```python
from build123d import *

# Parameters (mm, degrees)
SKETCH1_R           = 10.5
SKETCH1_R_2         = 9
BOSS_EXTRUDE1_DEPTH = 38.3
SKETCH2_R           = 1
SKETCH2_R_2         = 9
BOSS_EXTRUDE2_DEPTH = 1.5
FILLET1_R           = 0.5
SKETCH10_R          = 7.65
CUT_EXTRUDE1_DEPTH  = 46.293682625
SKETCH15_R          = 20.755300819
CUT_EXTRUDE3_DEPTH  = 17.5


with BuildPart() as part:
    # Sketch1 → Boss-Extrude1 (new body)
    with BuildSketch(Plane(origin=(0, 0, 0), x_dir=(1, 0, 0), z_dir=(0, 1, 0))):
        with Locations(Location((0, 0, 0), (0, 0, 270))):
            Circle(SKETCH1_R)
        with Locations(Location((0, 0, 0), (0, 0, 270))):
            Circle(SKETCH1_R_2, mode=Mode.SUBTRACT)
    extrude(amount=BOSS_EXTRUDE1_DEPTH)

    # Sketch2 → Boss-Extrude2 (add)
    with BuildSketch(Plane(origin=(0, 38.3, 0), x_dir=(1, 0, 0), z_dir=(0, 1, 0))):
        with BuildLine():
            Line((-3, -12.1346611), (-3, -12.5))
            ThreePointArc((-3, -12.5), (0, -15.5), (3, -12.5))
            Line((3, -12.5), (3, -12.1346611))
            ThreePointArc((3, -12.1346611), (6.25, -10.825317547), (9.008924778, -8.665406761))
            Line((9.008924778, -8.665406761), (9.325317547, -8.848076211))
            ThreePointArc((9.325317547, -8.848076211), (13.423393759, -7.75), (12.325317547, -3.651923789))
            Line((12.325317547, -3.651923789), (12.008924778, -3.469254338))
            ThreePointArc((12.008924778, -3.469254338), (12.393060767, -1.631577403), (12.497639685, 0.24290392))
            Line((12.497639685, 0.24290392), (12.850529964, 0.337460585))
            ThreePointArc((12.850529964, 0.337460585), (14.971850307, 4.011695199), (11.297615693, 6.133015543))
            Line((11.297615693, 6.133015543), (10.944725414, 6.038458877))
            ThreePointArc((10.944725414, 6.038458877), (7.609517863, 9.916916754), (3, 12.1346611))
            Line((3, 12.1346611), (3, 12.5))
            ThreePointArc((3, 12.5), (0, 15.5), (-3, 12.5))
            Line((-3, 12.5), (-3, 12.1346611))
            ThreePointArc((-3, 12.1346611), (-7.609517863, 9.916916754), (-10.944725414, 6.038458877))
            Line((-10.944725414, 6.038458877), (-11.297615693, 6.133015543))
            ThreePointArc((-11.297615693, 6.133015543), (-14.971850307, 4.011695199), (-12.850529964, 0.337460585))
            Line((-12.850529964, 0.337460585), (-12.497639685, 0.24290392))
            ThreePointArc((-12.497639685, 0.24290392), (-12.393060767, -1.631577403), (-12.008924778, -3.469254338))
            Line((-12.008924778, -3.469254338), (-12.325317547, -3.651923789))
            ThreePointArc((-12.325317547, -3.651923789), (-13.423393759, -7.75), (-9.325317547, -8.848076211))
            Line((-9.325317547, -8.848076211), (-9.008924778, -8.665406761))
            ThreePointArc((-9.008924778, -8.665406761), (-6.25, -10.825317547), (-3, -12.1346611))
        make_face()
        with Locations(Location((-12.074072829, 3.235238064, 0), (0, 0, 270))):
            Circle(SKETCH2_R, mode=Mode.SUBTRACT)
        with Locations(Location((0, 0, 0), (0, 0, 270))):
            Circle(SKETCH2_R_2, mode=Mode.SUBTRACT)
        with Locations((12.074072829, 3.235238064)):
            Circle(SKETCH2_R, mode=Mode.SUBTRACT)
        with Locations(Location((0, -12.5, 0), (0, 0, 270))):
            Circle(SKETCH2_R, mode=Mode.SUBTRACT)
    extrude(amount=BOSS_EXTRUDE2_DEPTH)

    # Fillet1
    fillet1_edges = [part.edges().sort_by_distance(p)[0] for p in [
        (-3, 39.05, 12.1346611),
        (3, 39.05, 12.1346611),
        (9.008924778, 39.05, 8.665406761),
        (12.008924778, 39.05, 3.469254338),
        (12.497639685, 39.05, -0.24290392),
        (10.944725414, 39.05, -6.038458877),
        (3, 39.05, -12.1346611),
        (-3, 39.05, -12.1346611),
        (-10.944725414, 39.05, -6.038458877),
        (-12.497639685, 39.05, -0.24290392),
        (-12.008924778, 39.05, 3.469254338),
        (-9.008924778, 39.05, 8.665406761),
    ]]
    fillet(fillet1_edges, radius=FILLET1_R)

    # Sketch10 → Cut-Extrude1 (cut, through all)
    with BuildSketch(Plane.XY):
        with Locations(Location((0, 10.55, 0), (0, 0, 90))):
            Circle(SKETCH10_R)
    extrude(amount=-CUT_EXTRUDE1_DEPTH, mode=Mode.SUBTRACT)

    # Sketch15 → Cut-Extrude3 (cut)
    with BuildSketch(Plane(origin=(0, 39.8, 0), x_dir=(1, 0, 0), z_dir=(0, 1, 0))):
        Circle(SKETCH15_R)
    extrude(amount=-CUT_EXTRUDE3_DEPTH, mode=Mode.SUBTRACT)


solid = part.part
```
Work out the finished part from the listing and answer in its coordinate system (mm). Give positions to 0.01 mm unless a question says otherwise; leave off trailing zeros. Loops run counter-clockwise (first coordinate to the right, second up) from the corner with the lowest first, then second, coordinate; pieces in that order, holes last. Notation, with made-up numbers: (21, 87.5) -> (56, 87.5) arc R15 ccw to (56, 99.5) -> close; hole circle Ø11 at (36.25, -35). An arc over 180 degrees is marked (long way). One line per question, with ' | ' between items. Start each with the question number.
1) Determine the mould class of faces 1 (the face through (3.2, 11, 10)), 2 (the face through (2.703, 10.994, 8.584)), 3 (the face through (8, 22.3, -5)), 4 (the face through (5.64, 15.72, -7.62)) for opening direction X: +X half, -X half, draft (parallel to the pull), parting line (faces both ways), or undercut.
2) Section A-A, the plane x = 0 is taken. Determine the outline of the cut face in (y, z).
3) Section C-C, the plane z = 8.5 is taken. Determine the outline of the cut face in (x, y).
4) Straight lines are drawn through the part: L1, parallel to X at y = 9.5, z = 0; L2, parallel to X at y = 5.75, z = -4.5; L3, parallel to Z at x = 4, y = 3.5. For each, find the intervals that lie inside material, in ascending order.
5) Section D-D, the plane y = 19.75 is taken. Determine the outline of the cut face in (x, z), then the cut area to 3 significant figures.
6) Section B-B, the plane z = 0 is taken. Determine the outline of the cut face in (x, y).
7) Each of these flat-tipped pins is pushed along its axis until it touches: pin 1 (6 mm diameter, centred on y = 12, z = -5.5, fed in from +X); pin 2 (10 mm diameter, centred on y = 5, z = -5.5, fed in from +X); pin 3 (4 mm diameter, centred on y = 4.5, z = 2.5, fed in from -X); pin 4 (4 mm diameter, centred on x = 5.5, z = 3.5, fed in from -Y). Where does it stop, or does it pass through?
Resolved:
1) face 1: parting line | face 2: undercut | face 3: draft | face 4: undercut
2) outline: (0, -10.5) -> (2.9, -10.5) -> (2.9, -9) -> (0, -9) -> close; (0, 9) -> (22.3, 9) -> (22.3, 10.5) -> (0, 10.5) -> close; (18.2, -10.5) -> (22.3, -10.5) -> (22.3, -9) -> (18.2, -9) -> close
3) outline: (-6.16, 0) -> (-2.96, 0) -> (-2.96, 22.3) -> (-6.16, 22.3) -> close; (2.96, 0) -> (6.16, 0) -> (6.16, 22.3) -> (2.96, 22.3) -> close
4) L1: -10.5 to -9, 9 to 10.5 | L2: -9.49 to -7.79, 7.79 to 9.49 | L3: -9.71 to -8.06, 8.06 to 9.71
5) outline: circle Ø21 at (0, 0); hole circle Ø18 at (0, 0) | area: 91.9 mm2
6) outline: (-10.5, 0) -> (-9, 0) -> (-9, 22.3) -> (-10.5, 22.3) -> close; (9, 0) -> (10.5, 0) -> (10.5, 22.3) -> (9, 22.3) -> close
7) pin 1: x = 10.2 | pin 2: x = 10.49 | pin 3: x = -10.49 | pin 4: through
